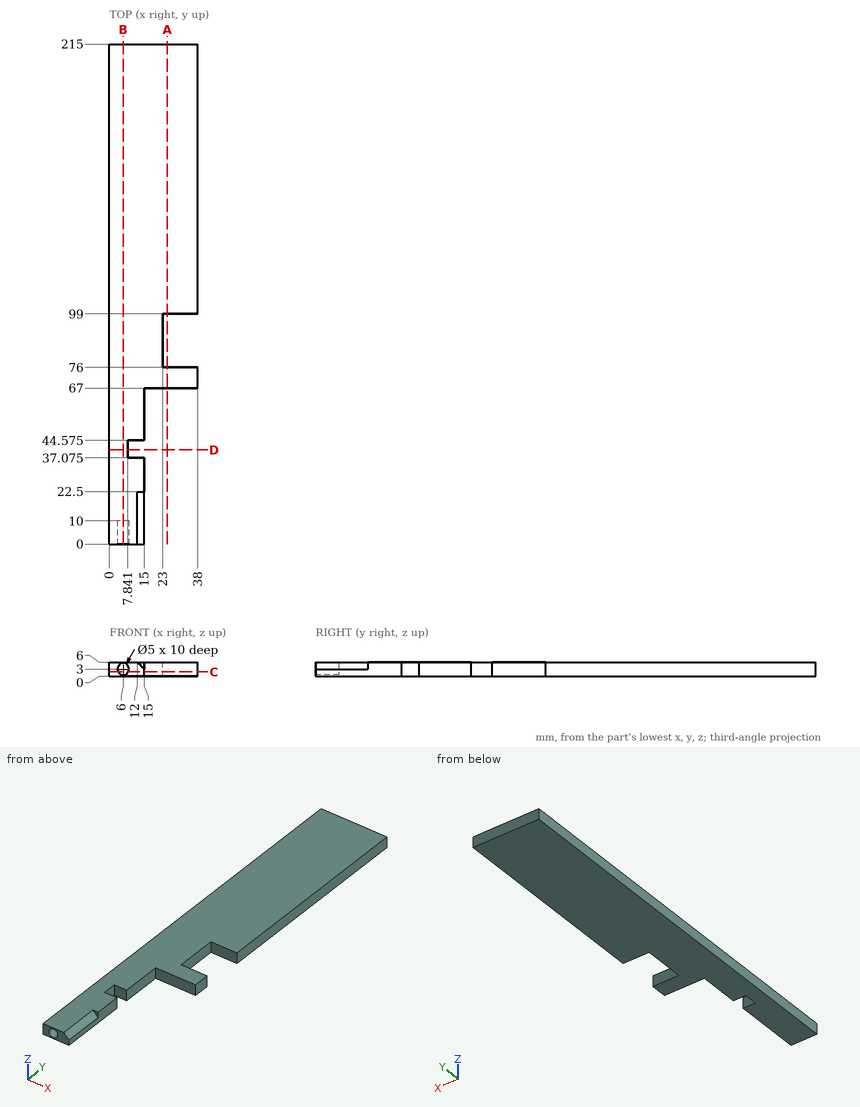
Here's the drawing with two shaded views (mm, measured from the low corner). I have some questions. Give positions to 0.01 mm unless a question says otherwise; leave off trailing zeros. Order: outer loops, then holes, each group sorted by start corner. A loop starts at its lowest first (then second) coordinate and runs counter-clockwise, first axis right, second up.
Q1. Suppose I cut it at D-D, the plane y = 40.5. Write out the boundary of the cut face in (x, z).
Q2. I'm going to push flat-ended pins straight in: P1, Ø1.8, axis at y = 41.5, z = 3, coming from the +X side; P2, Ø3, axis at y = 85, z = 4, coming from the +X side. Where does each tip first touch, or does it pass through?
Q3. Suppose I cut it at A-A, the plane x = 25. Write out the boundary of the cut face in (y, z), and give its area (3 significant figures).
Q4. If I drill on line 1 along Y through (x, z) = (33, 2); line 2 along Y through (x, z) = (10, 1.25) (1 decimal); line 3 along Z through (x, y) = (6, 7.5), over which ranges is the centre line in solid material (lowest first)?
Q5. Suppose I cut it at C-C, the plane z = 1.75. Write out the boundary of the cut face in (x, y) (1 decimal), and give its area (3 significant figures).
Q6. Suppose I cut it at B-B, the plane x = 6. Write out the boundary of the cut face in (y, z).
Solution:
1. outline: (0, 0) - (7.84, 0) - (7.84, 6) - (0, 6) - close
2. P1: stops at x = 7.84
2. P2: stops at x = 23
3. outline: (67, 0) - (76, 0) - (76, 6) - (67, 6) - close; (99, 0) - (215, 0) - (215, 6) - (99, 6) - close
3. area: 750 mm2
4. line 1: y = 67 to 76, 99 to 215
4. line 2: y = 0 to 37.1, 44.6 to 215
4. line 3: z = 0 to 0.5, 5.5 to 6
5. outline: (0, 0) - (3.8, 0) - (3.8, 10) - (8.2, 10) - (8.2, 0) - (15, 0) - (15, 37.1) - (7.8, 37.1) - (7.8, 44.6) - (15, 44.6) - (15, 67) - (38, 67) - (38, 76) - (23, 76) - (23, 99) - (38, 99) - (38, 215) - (0, 215) - close
5. area: 6,190 mm2
6. outline: (0, 0) - (215, 0) - (215, 6) - (0, 6) - (0, 5.5) - (10, 5.5) - (10, 0.5) - (0, 0.5) - close
